from build123d import *

# Parameters (mm, degrees)
PAD030_DEPTH         = 20
SKETCH094_R          = 2.5
POCKET048_DEPTH      = 42.001
POCKET048_DEPTH_BACK = 0.001
SKETCH095_R          = 2.63
POCKET049_DEPTH      = 30.001
POCKET049_DEPTH_BACK = 0.001
FILLET_R             = 3


with BuildPart() as part:
    # Sketch090 → Pad030 (new body)
    with BuildSketch(Plane(origin=(0, 92, 0), x_dir=(-1, 0, 0), z_dir=(0, 1, 0))):
        with BuildLine():
            Line((-13, 31), (-10.5, 31))
            Line((-10.5, 10.5), (-10.5, 31))
            Line((10.5, 10.5), (-10.5, 10.5))
            Line((10.5, 31), (10.5, 10.5))
            Line((10.5, 31), (13, 31))
            ThreePointArc((15, 29), (14.414214, 30.414214), (13, 31))
            Line((15, 29), (15, 9.872425))
            Line((10, -5.614149), (15, 9.872425))
            Line((10, -5.614149), (10, -11))
            Line((10, -11), (-10, -11))
            Line((-10, -11), (-10, -5.614149))
            Line((-10, -5.614149), (-15, 9.872425))
            Line((-15, 9.872425), (-15, 29))
            ThreePointArc((-13, 31), (-14.414214, 30.414214), (-15, 29))
        make_face()
    extrude(amount=-PAD030_DEPTH)

    # Sketch094 → Pocket048 (cut, two sides)
    with BuildSketch(Plane(origin=(0, 0, -11), x_dir=(-1, 0, 0), z_dir=(0, 0, -1))) as pocket048_sk:
        with Locations((0, 82)):
            Circle(SKETCH094_R)
    extrude(amount=-POCKET048_DEPTH, mode=Mode.SUBTRACT)
    extrude(pocket048_sk.sketch, amount=POCKET048_DEPTH_BACK, mode=Mode.SUBTRACT)

    # Sketch095 → Pocket049 (cut, two sides)
    with BuildSketch(Plane(origin=(15, 82, 0), x_dir=(0, 1, 0), z_dir=(1, 0, 0))) as pocket049_sk:
        with Locations((0, 22)):
            Circle(SKETCH095_R)
    extrude(amount=-POCKET049_DEPTH, mode=Mode.SUBTRACT)
    extrude(pocket049_sk.sketch, amount=POCKET049_DEPTH_BACK, mode=Mode.SUBTRACT)

    # Fillet
    fillet_edges = [part.edges().sort_by_distance(p)[0] for p in [
        (-12.5, 92, 2.129138),
        (-10, 92, -8.307075),
        (10, 92, -8.307075),
        (12.5, 92, 2.129138),
    ]]
    fillet(fillet_edges, radius=FILLET_R)


solid = part.part
Here's how the part is built. I have some questions about the finished solid (model axes, mm). A direction names the side the tool comes from. Coordinates: 2 decimals unless noted, no trailing zeros. Order: outer loops, then holes, each group sorted by start corner. A loop starts at its lowest first (then second) coordinate and runs counter-clockwise, first axis right, second up. Notation, with made-up numbers: (23, -5) -> (45, -5) arc R23 cw to (45, 24) -> close; hole circle Ø3 at (40, 88). An arc over 180 degrees is marked (long way). Answer in a Markdown table with one row per item.
(1) On a 3-axis mill with a long thin cutter (end or side, diameter ignored), from which of +Z, -Z, +X, -X, +Y, -Y can I reach the whole of each face in a straight line? I mean faces 5 (the face through (-14.43, 82.14, 30.4)), 6 (the face through (-10.5, 82, 19)), 7 (the face through (-10, 81, -8)). Say none if no direction works.
Answer key:
| item | result |
|---|---|
| face 5 | +Z, -X, +Y, -Y |
| face 6 | +Z, +Y, -Y |
| face 7 | -Z, -X, +Y, -Y |
(2) I want a section at C-C on y = 88.5. List the corners of the cut face in (x, z) for me, then the cut area to 3 significant figures.
Answer key:
| item | result |
|---|---|
| outline | (-15, 9.87) -> (-10, -5.61) -> (-10, -11) -> (10, -11) -> (10, -5.61) -> (15, 9.87) -> (15, 29) arc R2 ccw to (13, 31) -> (10.5, 31) -> (10.5, 10.5) -> (-10.5, 10.5) -> (-10.5, 31) -> (-13, 31) arc R2 ccw to (-15, 29) -> close |
| area | 696 mm^2 |
(3) I want a section at D-D on x = -1. List the corners of the cut face in (y, z) for me, then the cut area to 3 significant figures.
Answer key:
| item | result |
|---|---|
| outline | (72, -11) -> (79.71, -11) -> (79.71, 10.5) -> (72, 10.5) -> close; (84.29, -11) -> (92, -11) -> (92, 10.5) -> (84.29, 10.5) -> close |
| area | 331 mm^2 |
(4) I want a section at A-A on y = 82. List the corners of the cut face in (x, z) for me.
Answer key:
| item | result |
|---|---|
| outline | (-15, 9.87) -> (-10, -5.61) -> (-10, -11) -> (-2.5, -11) -> (-2.5, 10.5) -> (-10.5, 10.5) -> (-10.5, 19.37) -> (-15, 19.37) -> close; (-15, 24.63) -> (-10.5, 24.63) -> (-10.5, 31) -> (-13, 31) arc R2 ccw to (-15, 29) -> close; (2.5, -11) -> (10, -11) -> (10, -5.61) -> (15, 9.87) -> (15, 19.37) -> (10.5, 19.37) -> (10.5, 10.5) -> (2.5, 10.5) -> close; (10.5, 24.63) -> (15, 24.63) -> (15, 29) arc R2 ccw to (13, 31) -> (10.5, 31) -> close |
(5) Thinking about a two-plate mould opening in Z: for faces 1 (the face through (12, 82, 31)), 2 (the face through (12.2, 91.1, 4)), 3 (the face through (9.1, 91.14, -8.03)), 4 (the face through (-12.72, 84.43, 20.99)), which applies, +Z half, -Z half, draft (parallel to the pull), parting line (faces both ways), or undercut?
Answer key:
| item | result |
|---|---|
| face 1 | +Z half |
| face 2 | -Z half |
| face 3 | draft |
| face 4 | undercut |
(6) Please list where these lines run through material, in increasing order: probe 1 along X at (y, z) = (91, 18); probe 2 along Y at (x, z) = (0, 0.5); probe 3 along Z at (x, y) = (8, 83.25).
Answer key:
| item | result |
|---|---|
| probe 1 | -15 to -10.5, 10.5 to 15 |
| probe 2 | 72 to 79.5, 84.5 to 92 |
| probe 3 | -11 to 10.5 |
(7) Will these pins go through, and if not, where does the flat tip stop? pin 1 Ø1.6 at (y, z) = (81.5, -9) entering from -X; pin 2 Ø6 at (x, y) = (1, 80) entering from +Z; pin 3 Ø5 at (y, z) = (78, 7) entering from +X.
Answer key:
| item | result |
|---|---|
| pin 1 | x = -10 |
| pin 2 | z = 10.5 |
| pin 3 | x = 14.88 |
(8) I want a section at B-B on z = 22. List the corners of the cut face in (x, y) for me, then the cut area to 3 significant figures.
Answer key:
| item | result |
|---|---|
| outline | (-15, 72) -> (-10.5, 72) -> (-10.5, 79.37) -> (-15, 79.37) -> close; (-15, 84.63) -> (-10.5, 84.63) -> (-10.5, 92) -> (-15, 92) -> close; (10.5, 72) -> (15, 72) -> (15, 79.37) -> (10.5, 79.37) -> close; (10.5, 84.63) -> (15, 84.63) -> (15, 92) -> (10.5, 92) -> close |
| area | 133 mm^2 |
